```python
from build123d import *

# Parameters (mm, degrees)
ESBO_O1_R                     = 2
ESBO_O1_W                     = 10
ESBO_O1_H                     = 16
ESBO_O1_H_2                   = 2
RESSALTO_EXTRUS_O1_DEPTH      = 3
ESBO_O1_4_W                   = 10
ESBO_O1_4_H                   = 2
RESSALTO_EXTRUS_O5_DEPTH      = 15.5
RESSALTO_EXTRUS_O6_DEPTH      = 12.5
ESBO_O11_W                    = 2
ESBO_O11_H                    = 12.5
RESSALTO_EXTRUS_O7_DEPTH      = 11
RESSALTO_EXTRUS_O8_DEPTH      = 18
ESBO_O8_W                     = 14.4
ESBO_O8_H                     = 12.5
CORTE_EXTRUS_O1_DEPTH         = 40.764934301
FILETE1_R                     = 5
RESSALTO_EXTRUS_O9_DEPTH      = 2
RESSALTO_EXTRUS_O9_DEPTH_BACK = 18
ESBO_O18_W                    = 6
ESBO_O18_H                    = 16
CORTE_EXTRUS_O3_DEPTH         = 35.311076929


with BuildPart() as part:
    # Esboço1 → Ressalto-extrusão1 (new body)
    # profile 1 of 9: a face of its own
    with BuildSketch(Plane(origin=(0, 0, 0), x_dir=(1, 0, 0), z_dir=(0, 1, 0))):
        Polygon((10, 5), (-6.376571145, 5), (-6.376571145, -0.435143283), (-3.333333333, -5), (10, -5), align=None)
        with Locations(Location((1.811714428, -0.905857214, 0), (0, 0, 270))):
            Circle(ESBO_O1_R, mode=Mode.SUBTRACT)
    # profile 2 of 9: a face of its own
    with BuildSketch(Plane(origin=(0, 0, 0), x_dir=(1, 0, 0), z_dir=(0, 1, 0))):
        Polygon((10, -5), (-3.333333333, -5), (0, -10), (5, -10), (10, -10), align=None)
    # profile 3 of 9: a face of its own
    with BuildSketch(Plane(origin=(0, 0, 0), x_dir=(1, 0, 0), z_dir=(0, 1, 0))):
        Polygon((10, -5), (-3.333333333, -5), (0, -10), (5, -10), (10, -10), align=None)
    # profile 4 of 9: a face of its own
    with BuildSketch(Plane(origin=(0, 0, 0), x_dir=(1, 0, 0), z_dir=(0, 1, 0))):
        Polygon((10, -5), (-3.333333333, -5), (0, -10), (5, -10), (10, -10), align=None)
    # profile 5 of 9: a face of its own
    with BuildSketch(Plane(origin=(0, 0, 0), x_dir=(1, 0, 0), z_dir=(0, 1, 0))):
        Polygon((10, -5), (-3.333333333, -5), (0, -10), (5, -10), (10, -10), align=None)
    # profile 6 of 9: a face of its own
    with BuildSketch(Plane(origin=(0, 0, 0), x_dir=(1, 0, 0), z_dir=(0, 1, 0))):
        with Locations((5, -20)):
            Rectangle(ESBO_O1_W, ESBO_O1_H)
    # profile 7 of 9: a face of its own
    with BuildSketch(Plane(origin=(0, 0, 0), x_dir=(1, 0, 0), z_dir=(0, 1, 0))):
        with Locations((5, -29)):
            Rectangle(ESBO_O1_W, ESBO_O1_H_2)
    # profile 8 of 9: a face of its own
    with BuildSketch(Plane(origin=(0, 0, 0), x_dir=(1, 0, 0), z_dir=(0, 1, 0))):
        with Locations((5, -20)):
            Rectangle(ESBO_O1_W, ESBO_O1_H)
    # profile 9 of 9: a face of its own
    with BuildSketch(Plane(origin=(0, 0, 0), x_dir=(1, 0, 0), z_dir=(0, 1, 0))):
        Polygon((5, -10), (0, -10), (0, -12), (10, -12), (10, -10), align=None)
    extrude(amount=RESSALTO_EXTRUS_O1_DEPTH)

    # Esboço1<4> → Ressalto-extrusão5 (add)
    with BuildSketch(Plane(origin=(0, 0, 0), x_dir=(1, 0, 0), z_dir=(0, 1, 0))):
        with Locations((5, -11)):
            Rectangle(ESBO_O1_4_W, ESBO_O1_4_H)
        with Locations((5, -29)):
            Rectangle(ESBO_O1_4_W, ESBO_O1_4_H)
    extrude(amount=RESSALTO_EXTRUS_O5_DEPTH)

    # Esboço10 → Ressalto-extrusão6 (add)
    with BuildSketch(Plane(origin=(0, 3, 0), x_dir=(1, 0, 0), z_dir=(0, 1, 0))):
        Polygon((-2.729428524, -5.905857214), (0, -10), (10, -10), (10, -5.905857214), (1.811714428, -5.905857214), (0, -5.905857214), align=None)
    extrude(amount=RESSALTO_EXTRUS_O6_DEPTH)

    # Esboço11 → Ressalto-extrusão7 (add)
    with BuildSketch(Plane.ZY):
        with Locations((11, 9.25)):
            Rectangle(ESBO_O11_W, ESBO_O11_H)
        with Locations((29, 9.25)):
            Rectangle(ESBO_O11_W, ESBO_O11_H)
    extrude(amount=RESSALTO_EXTRUS_O7_DEPTH)

    # Esboço12 → Ressalto-extrusão8 (add)
    with BuildSketch(Plane.XY.offset(30)):
        with BuildLine():
            ThreePointArc((-6.656098816, 10.563748655), (-7.25, 9.25), (-6.656098816, 7.936251345))
            Line((-6.656098816, 7.936251345), (-5.5, 9.25))
            Line((-5.5, 9.25), (-6.656098816, 10.563748655))
        make_face()
        with BuildLine():
            Line((-5.5, 9.25), (-6.656098816, 7.936251345))
            ThreePointArc((-6.656098816, 7.936251345), (-5.5, 7.5), (-4.343901184, 7.936251345))
            Line((-4.343901184, 7.936251345), (-5.5, 9.25))
        make_face()
        with BuildLine():
            Line((-6.656098816, 10.563748655), (-5.5, 9.25))
            Line((-5.5, 9.25), (-4.343901184, 10.563748655))
            ThreePointArc((-4.343901184, 10.563748655), (-5.5, 11), (-6.656098816, 10.563748655))
        make_face()
        with BuildLine():
            Line((-4.343901184, 10.563748655), (-5.5, 9.25))
            Line((-5.5, 9.25), (-4.343901184, 7.936251345))
            ThreePointArc((-4.343901184, 7.936251345), (-3.905372625, 8.529123079), (-3.75, 9.25))
            ThreePointArc((-3.75, 9.25), (-3.905372625, 9.970876921), (-4.343901184, 10.563748655))
        make_face()
    extrude(amount=-RESSALTO_EXTRUS_O8_DEPTH)

    # Esboço8 → Corte-extrusão1 (cut, through all)
    with BuildSketch(Plane(origin=(10, 0, 0), x_dir=(0, 0, -1), z_dir=(1, 0, 0))):
        with Locations((-20, 9.25)):
            Rectangle(ESBO_O8_W, ESBO_O8_H)
    extrude(amount=-CORTE_EXTRUS_O1_DEPTH, mode=Mode.SUBTRACT)

    # Filete1
    filete1_edges = [part.edges().sort_by_distance(p)[0] for p in [
        (-11, 15.5, 11),
        (-11, 3, 11),
        (-11, 3, 29),
        (-11, 15.5, 29),
    ]]
    fillet(filete1_edges, radius=FILETE1_R)

    # Esboço14 → Ressalto-extrusão9 (add, two sides: drawn at the far end of the back side and taken through both)
    with BuildSketch(Plane(origin=(0, 3, 28), x_dir=(1, 0, 0), z_dir=(0, 0, 1)).offset(-RESSALTO_EXTRUS_O9_DEPTH_BACK)):
        Polygon((0, -3), (-2.25, 0), (-5.913171112, 0), align=None)
        Polygon((0, 0), (-2.25, 0), (0, -3), align=None)
    extrude(amount=RESSALTO_EXTRUS_O9_DEPTH + RESSALTO_EXTRUS_O9_DEPTH_BACK)

    # Esboço18 → Corte-extrusão3 (cut, through all)
    with BuildSketch(Plane(origin=(0, 3, 0), x_dir=(1, 0, 0), z_dir=(0, 1, 0))):
        with Locations((-2.913171112, -20)):
            Rectangle(ESBO_O18_W, ESBO_O18_H)
    extrude(amount=-CORTE_EXTRUS_O3_DEPTH, mode=Mode.SUBTRACT)


solid = part.part
```
The model under review builds one solid part; all positions refer to its coordinate system, in mm. A direction names the side the tool comes from. Round coordinates to 2 decimals unless told otherwise and drop trailing zeros. Loops run counter-clockwise (first coordinate to the right, second up) from the corner with the lowest first, then second, coordinate; pieces in that order, holes last. Notation, with made-up numbers: (84, 54.5) - (94, 54.5) arc R24 cw to (94, 75.5) - close; hole circle Ø10 at (12.25, -9.5). An arc over 180 degrees is marked (long way). Use a Markdown table: item, result. Add a question column.
Q1. For probe 1 along Z at (x, y) = (-6.5, 5.5); probe 2 along Z at (x, y) = (6.75, 10.75); probe 3 along X at (y, z) = (1.75, 16.5), list the stretches that pass through material, from the lowest coordinate up.
Q2. Insertion check: pin 1 Ø5 at (y, z) = (4.5, 24.5) entering from -X; pin 2 Ø6 at (x, z) = (-7, 7.5) entering from -Y; pin 3 Ø8 at (x, y) = (2, 11) entering from -Z; pin 4 Ø2.5 at (x, z) = (1.81, 0.91) entering from +Y. Each pin has a flat end and moves straight along its axis. Give the tip position at first contact, or say it passes through.
Q3. Add section D-D (z = 11.5). State the section outline as (x, y) points.
Q4. Add section A-A (y = 9.75). State the section outline as (x, z) points, plus the area to 3 significant figures.
Q5. Add section B-B (x = 0.5). State the section outline as (y, z) points, plus the area to 3 significant figures.
Q6. Machinability: for faces 1 (the face through (-3, 1.52, 10.99)), 2 (the face through (-5, 9, 27.2)), 3 (the face through (5, 3, 20)), which of the approach directions +Z, -Z, +X, -X, +Y, -Y give a long, thin tool a straight path to every point of the face, cutting with its end or side? Answer none if there is none.
Q7. The part is to be moulded in two halves that separate along X. For faces 4 (the face through (4, 15.5, 9)), 5 (the face through (0.087, 2, 20)), 6 (the face through (3.795, 1.479, 0.645)), say which applies: pulls with the +X half, pulls with the -X half, needs draft (parallel to the pull), parting line crosses it, or undercut.
Q8. Add section C-C (x = 8.5). State the section outline as (y, z) points, plus the area to 3 significant figures.
Worked answers:
| question | item | result |
|---|---|---|
| 1 | probe 1 | 10 to 12, 28 to 30 |
| 1 | probe 2 | 5.91 to 12, 28 to 30 |
| 1 | probe 3 | 0.09 to 10 |
| 2 | pin 1 | x = 0.09 |
| 2 | pin 2 | y = 2.71 |
| 2 | pin 3 | z = 5.91 |
| 2 | pin 4 | through |
| 3 | outline | (-11, 8) arc R5 ccw to (-6, 3) - (-5.91, 3) - (0, 0) - (10, 0) - (10, 15.5) - (-6, 15.5) arc R5 ccw to (-11, 10.5) - close |
| 4 | outline | (-11, 10) - (0, 10) - (-2.73, 5.91) - (10, 5.91) - (10, 12) - (-3.82, 12) - (-3.82, 12.8) - (-7.18, 12.8) - (-7.18, 12) - (-11, 12) - close; (-11, 28) - (-7.18, 28) - (-7.18, 27.2) - (-3.82, 27.2) - (-3.82, 28) - (10, 28) - (10, 30) - (-11, 30) - close |
| 4 | area | 136 mm² |
| 5 | outline | (0, -5) - (3, -5) - (3, -0.6) - (0, -0.6) - close; (0, 2.42) - (3, 2.42) - (3, 5.91) - (15.5, 5.91) - (15.5, 12) - (3, 12) - (3, 28) - (15.5, 28) - (15.5, 30) - (0, 30) - close |
| 5 | area | 197 mm² |
| 6 | face 1 | +Z, -X, -Y |
| 6 | face 2 | +X, -X, +Y, -Y |
| 6 | face 3 | +X, -X, +Y |
| 7 | face 4 | needs draft |
| 7 | face 5 | pulls with the -X half |
| 7 | face 6 | undercut |
| 8 | outline | (0, -5) - (3, -5) - (3, 5.91) - (15.5, 5.91) - (15.5, 12) - (3, 12) - (3, 28) - (15.5, 28) - (15.5, 30) - (0, 30) - close |
| 8 | area | 206 mm² |
